Geometry check sheet. Reference: the model listing, model coordinates, mm. Coordinates: 2 decimals unless noted, no trailing zeros. Write each loop counter-clockwise with the first axis right and the second up, starting at its lowest first coordinate (ties: lowest second). Pieces come first, ordered by that corner, then holes. Notation, with made-up numbers: (88, 32.25) -> (112, 32.25) arc R29 cw to (112, 68.25) -> close; hole circle Ø8 at (62, 27). An arc over 180 degrees is marked (long way). Use a Markdown table: item, result.
```python
from build123d import *

# Parameters (mm, degrees)
F0_W     = 140
F0_H     = 50
F0_R     = 3.5
F0_R_2   = 2
F0_R_3   = 2.75
F0_R_4   = 9.25
F0_R_5   = 6
F0_R_6   = 11
F1_DEPTH = 8
F2_D     = 4
F3_SIZE  = 3


with BuildPart() as f1:
    # F0 (on Front) → F1 (new body)
    with BuildSketch(Plane.XZ):
        with Locations((70, 25)):
            Rectangle(F0_W, F0_H)
        with Locations((7.5, 7.5)):
            Circle(F0_R, mode=Mode.SUBTRACT)
        with Locations((29.686291501, 13.686291501)):
            Circle(F0_R_2, mode=Mode.SUBTRACT)
        with Locations((52.313708499, 13.686291501)):
            Circle(F0_R_2, mode=Mode.SUBTRACT)
        with Locations((63, 18)):
            Circle(F0_R_3, mode=Mode.SUBTRACT)
        with Locations((132.5, 7.5)):
            Circle(F0_R, mode=Mode.SUBTRACT)
        with Locations((77, 18)):
            Circle(F0_R_3, mode=Mode.SUBTRACT)
        with Locations((87.686291501, 13.686291501)):
            Circle(F0_R_2, mode=Mode.SUBTRACT)
        with Locations((110.313708499, 13.686291501)):
            Circle(F0_R_2, mode=Mode.SUBTRACT)
        with Locations((29.686291501, 36.313708499)):
            Circle(F0_R_2, mode=Mode.SUBTRACT)
        with Locations((41, 25)):
            Circle(F0_R_4, mode=Mode.SUBTRACT)
        with Locations((52.313708499, 36.313708499)):
            Circle(F0_R_2, mode=Mode.SUBTRACT)
        with Locations((63, 32)):
            Circle(F0_R_3, mode=Mode.SUBTRACT)
        with Locations((7.5, 42.5)):
            Circle(F0_R, mode=Mode.SUBTRACT)
        with Locations((70, 25)):
            Circle(F0_R_5, mode=Mode.SUBTRACT)
        with Locations((99, 25)):
            Circle(F0_R_6, mode=Mode.SUBTRACT)
        with Locations((77, 32)):
            Circle(F0_R_3, mode=Mode.SUBTRACT)
        with Locations((87.686291501, 36.313708499)):
            Circle(F0_R_2, mode=Mode.SUBTRACT)
        with Locations((110.313708499, 36.313708499)):
            Circle(F0_R_2, mode=Mode.SUBTRACT)
        with Locations((132.5, 42.5)):
            Circle(F0_R, mode=Mode.SUBTRACT)
        with Locations((52.313708499, 36.313708499)):
            Circle(F0_R_2)
        with Locations((29.686291501, 36.313708499)):
            Circle(F0_R_2)
        with Locations((29.686291501, 13.686291501)):
            Circle(F0_R_2)
        with Locations((52.313708499, 13.686291501)):
            Circle(F0_R_2)
        with Locations((87.686291501, 13.686291501)):
            Circle(F0_R_2)
        with Locations((110.313708499, 13.686291501)):
            Circle(F0_R_2)
        with Locations((110.313708499, 36.313708499)):
            Circle(F0_R_2)
        with Locations((87.686291501, 36.313708499)):
            Circle(F0_R_2)
    extrude(amount=F1_DEPTH)

    # F2 (through all)
    with Locations(Plane(origin=(0, 0, 0), x_dir=(1, 0, 0), z_dir=(0, 1, 0))):
        with Locations((29.686291501, -36.313708499), (29.686291501, -13.686291501), (52.313708499, -13.686291501), (52.313708499, -36.313708499), (87.686291501, -36.313708499), (87.686291501, -13.686291501), (110.313708499, -13.686291501), (110.313708499, -36.313708499)):
            Hole(F2_D / 2)

    # F3
    f3_edges = [f1.edges().sort_by_distance(p)[0] for p in [
        (140, -4, 50),
        (140, -4, 0),
        (0, -4, 0),
        (0, -4, 50),
    ]]
    chamfer(f3_edges, length=F3_SIZE)


solid = f1.part
```
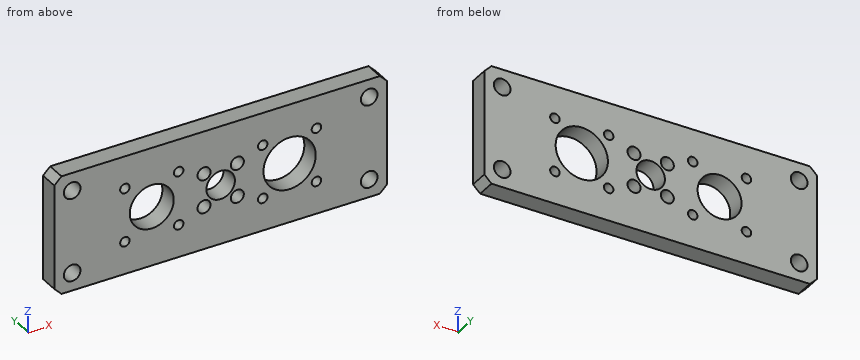
Item 1: Depth check by flat-ended pin: P1, Ø8, axis at x = 132.5, z = 42.5, coming from the +Y side; P2, Ø3.5, axis at x = 52.31, z = 36.31, coming from the +Y side. Enter the tip coordinate at first touch or a pass-through.
Answer block:
| item | result |
|---|---|
| P1 | stops at y = 0 |
| P2 | passes through |
Item 2: Thickness scan on L1, parallel to Z at x = 63, y = -5; L2, parallel to X at y = -3.5, z = 24.5; L3, parallel to X at y = -4.5, z = 27. Record the ranges inside material, lowest first. Write a range as [from, to].
Answer block:
| item | result |
|---|---|
| L1 | z = [0, 15.25], [20.75, 29.25], [34.75, 50] |
| L2 | x = [0, 31.76], [50.24, 64.02], [75.98, 88.01], [109.99, 140] |
| L3 | x = [0, 31.97], [50.03, 64.34], [75.66, 88.18], [109.82, 140] |
Item 3: Section check C-C on x = 61.5. Record the boundary of the cut face in (y, z), then the cut area to 3 significant figures.
Answer block:
| item | result |
|---|---|
| outline | (-8, 0) -> (0, 0) -> (0, 15.7) -> (-8, 15.7) -> close; (-8, 20.3) -> (0, 20.3) -> (0, 29.7) -> (-8, 29.7) -> close; (-8, 34.3) -> (0, 34.3) -> (0, 50) -> (-8, 50) -> close |
| area | 326 mm^2 |
Item 4: Section check A-A on x = 41. Record the boundary of the cut face in (y, z).
Answer block:
| item | result |
|---|---|
| outline | (-8, 0) -> (0, 0) -> (0, 15.75) -> (-8, 15.75) -> close; (-8, 34.25) -> (0, 34.25) -> (0, 50) -> (-8, 50) -> close |
Item 5: Section check B-B on z = 7.5. Record the boundary of the cut face in (x, y).
Answer block:
| item | result |
|---|---|
| outline | (0, -8) -> (4, -8) -> (4, 0) -> (0, 0) -> close; (11, -8) -> (129, -8) -> (129, 0) -> (11, 0) -> close; (136, -8) -> (140, -8) -> (140, 0) -> (136, 0) -> close |
Item 6: Section check D-D on y = -4. Count the separate pieces of the cut face and the enclosed holes in it, then the cut area to 3 significant figures.
Answer block:
| item | result |
|---|---|
| separate pieces | 1 |
| enclosed holes | 19 |
| area | 5,870 mm^2 |
